For this review, take the finished solid that the model builds, in its own axes (mm). Coordinates: 2 decimals unless noted, no trailing zeros. Loops run counter-clockwise (first coordinate to the right, second up) from the corner with the lowest first, then second, coordinate; pieces in that order, holes last. Notation, with made-up numbers: (-28.75, 21) -> (24.25, 21) arc R21 ccw to (24.25, 57) -> close; hole circle Ø5 at (-21, 84). An arc over 180 degrees is marked (long way). Answer in a Markdown table with one row per item.
from build123d import *

# Parameters (mm, degrees)
SKETCH_1_W                         = 25.9
SKETCH_1_H                         = 2.5
EXTRUDE_1_DEPTH                    = 8.5
SKETCH_2_W                         = 0.5
SKETCH_2_H                         = 0.5
CUT_EXTRUDE_1_DEPTH                = 7.5
CHAMFER_1_SIZE                     = 0.75
SKETCH_6_W                         = 0.5
SKETCH_6_H                         = 0.5
CUT_EXTRUDE_3_DEPTH                = 7.5
CHAMFER_3_SIZE                     = 0.75
PATTERN_LINEAR_1_COUNT             = 5
PATTERN_LINEAR_1_PITCH             = 2.54
CHAMFER_3_OF_PATTERN_LINEAR_1_SIZE = 0.75
PATTERN_LINEAR_2_COUNT             = 5
PATTERN_LINEAR_2_PITCH             = 2.54
CHAMFER_1_OF_PATTERN_LINEAR_2_SIZE = 0.75


with BuildPart() as part:
    # Эскиз1 → Бобышка-Вытянуть1 (new body)
    with BuildSketch(Plane(origin=(0, 0, 0), x_dir=(1, 0, 0), z_dir=(0, 1, 0))):
        Rectangle(SKETCH_1_W, SKETCH_1_H)
    extrude(amount=EXTRUDE_1_DEPTH)

    # Эскиз2 → Вырез-Вытянуть1 (cut)
    with BuildSketch(Plane(origin=(0, 8.5, 0), x_dir=(1, 0, 0), z_dir=(0, 1, 0))):
        with Locations((1.27, 0)):
            Rectangle(SKETCH_2_W, SKETCH_2_H)
    cut_extrude_1 = extrude(amount=-CUT_EXTRUDE_1_DEPTH, mode=Mode.SUBTRACT)

    # Фаска1
    chamfer_1_edges = [part.edges().sort_by_distance(p)[0] for p in [
        (1.52, 8.5, 0),
        (1.27, 8.5, -0.25),
        (1.02, 8.5, 0),
        (1.27, 8.5, 0.25),
    ]]
    chamfer(chamfer_1_edges, length=CHAMFER_1_SIZE)

    # Эскиз6 → Вырез-Вытянуть3 (cut)
    with BuildSketch(Plane(origin=(0, 8.5, 0), x_dir=(1, 0, 0), z_dir=(0, 1, 0))):
        with Locations((-1.27, 0)):
            Rectangle(SKETCH_6_W, SKETCH_6_H)
    cut_extrude_3 = extrude(amount=-CUT_EXTRUDE_3_DEPTH, mode=Mode.SUBTRACT)

    # Фаска3
    chamfer_3_edges = [part.edges().sort_by_distance(p)[0] for p in [
        (-1.02, 8.5, 0),
        (-1.27, 8.5, -0.25),
        (-1.52, 8.5, 0),
        (-1.27, 8.5, 0.25),
    ]]
    chamfer(chamfer_3_edges, length=CHAMFER_3_SIZE)

    # Линейный массив1: Вырез-Вытянуть3 ×5
    with Locations(*[(-i * PATTERN_LINEAR_1_PITCH, 0, 0) for i in range(1, PATTERN_LINEAR_1_COUNT)]):
        add(cut_extrude_3, mode=Mode.SUBTRACT)

    # Фаска3 of Линейный массив1
    chamfer_3_of_pattern_linear_1_edges = [part.edges().sort_by_distance(p)[0] for p in [
        (-3.56, 8.5, 0),
        (-3.81, 8.5, -0.25),
        (-4.06, 8.5, 0),
        (-3.81, 8.5, 0.25),
        (-6.1, 8.5, 0),
        (-6.35, 8.5, -0.25),
        (-6.6, 8.5, 0),
        (-6.35, 8.5, 0.25),
        (-8.64, 8.5, 0),
        (-8.89, 8.5, -0.25),
        (-9.14, 8.5, 0),
        (-8.89, 8.5, 0.25),
        (-11.18, 8.5, 0),
        (-11.43, 8.5, -0.25),
        (-11.68, 8.5, 0),
        (-11.43, 8.5, 0.25),
    ]]
    chamfer(chamfer_3_of_pattern_linear_1_edges, length=CHAMFER_3_OF_PATTERN_LINEAR_1_SIZE)

    # Линейный массив2: Вырез-Вытянуть1 ×5
    with Locations(*[(i * PATTERN_LINEAR_2_PITCH, 0, 0) for i in range(1, PATTERN_LINEAR_2_COUNT)]):
        add(cut_extrude_1, mode=Mode.SUBTRACT)

    # Фаска1 of Линейный массив2
    chamfer_1_of_pattern_linear_2_edges = [part.edges().sort_by_distance(p)[0] for p in [
        (4.06, 8.5, 0),
        (3.81, 8.5, -0.25),
        (3.56, 8.5, 0),
        (3.81, 8.5, 0.25),
        (6.6, 8.5, 0),
        (6.35, 8.5, -0.25),
        (6.1, 8.5, 0),
        (6.35, 8.5, 0.25),
        (9.14, 8.5, 0),
        (8.89, 8.5, -0.25),
        (8.64, 8.5, 0),
        (8.89, 8.5, 0.25),
        (11.68, 8.5, 0),
        (11.43, 8.5, -0.25),
        (11.18, 8.5, 0),
        (11.43, 8.5, 0.25),
    ]]
    chamfer(chamfer_1_of_pattern_linear_2_edges, length=CHAMFER_1_OF_PATTERN_LINEAR_2_SIZE)


solid = part.part
Item 1: Take a section at B-B, the plane y = 1.75. Count the separate pieces of the cut face and the enclosed holes in it, and give its area (4 significant figures).
Worked answers:
| item | result |
|---|---|
| separate pieces | 1 |
| enclosed holes | 10 |
| area | 62.25 mm² |
Item 2: Take a section at C-C, the plane x = 8.25. State the section outline as (y, z) points.
Worked answers:
| item | result |
|---|---|
| outline | (0, -1.25) -> (8.5, -1.25) -> (8.5, -1) -> (8.14, -0.64) -> (8.14, 0.64) -> (8.5, 1) -> (8.5, 1.25) -> (0, 1.25) -> close |
Item 3: For L1, parallel to Z at x = -1.25, y = 2.5; L2, parallel to Z at x = 3.5, y = 8; L3, parallel to Y at x = -4, z = 0.2, list the stretches that pass through material, from the lowest coordinate up.
Worked answers:
| item | result |
|---|---|
| L1 | -1.25 to -0.25, 0.25 to 1.25 |
| L2 | -1.25 to -0.5, 0.5 to 1.25 |
| L3 | 0 to 1 |
Item 4: Take a section at A-A, the plane x = 1.25. State the section outline as (y, z) points.
Worked answers:
| item | result |
|---|---|
| outline | (0, -1.25) -> (8.5, -1.25) -> (8.5, -1) -> (7.75, -0.25) -> (1, -0.25) -> (1, 0.25) -> (7.75, 0.25) -> (8.5, 1) -> (8.5, 1.25) -> (0, 1.25) -> close |
